from build123d import *

# Parameters (mm, degrees)
SKETCH1_W               = 96
SKETCH1_H               = 185
PLATE_DEPTH             = 5
STANDOFF_HOLES_REACH    = 106.332
SKETCH2_R               = 1.7
POWER_BOARD_HOLES_REACH = 106.332
SKETCH3_R               = 1.7
FILLET1_R               = 1
M2_5_CLEARANCE_HOLE1_D  = 2.9
M3_CLEARANCE_HOLE2_D    = 3.4
CUT_EXTRUDE1_REACH      = 106.332


with BuildPart() as part:
    # Sketch1 → plate (new body)
    with BuildSketch(Plane(origin=(0, 0, 0), x_dir=(1, 0, 0), z_dir=(0, 1, 0))):
        Rectangle(SKETCH1_W, SKETCH1_H)
    extrude(amount=PLATE_DEPTH)

    # Sketch2 → standoff-holes (cut, up to next)
    with BuildSketch(Plane(origin=(0, 5, 0), x_dir=(1, 0, 0), z_dir=(0, 1, 0)), mode=Mode.PRIVATE) as standoff_holes_sk1:
        with Locations(Location((44, 74, 0), (0, 0, 270))):
            Circle(SKETCH2_R)
    standoff_holes_tool1 = extrude(standoff_holes_sk1.sketch, amount=-STANDOFF_HOLES_REACH, mode=Mode.PRIVATE) & part.part
    # Sketch2 → standoff-holes (cut, up to next)
    with BuildSketch(Plane(origin=(0, 5, 0), x_dir=(1, 0, 0), z_dir=(0, 1, 0)), mode=Mode.PRIVATE) as standoff_holes_sk2:
        with Locations(Location((-44, 74, 0), (0, 0, 270))):
            Circle(SKETCH2_R)
    standoff_holes_tool2 = extrude(standoff_holes_sk2.sketch, amount=-STANDOFF_HOLES_REACH, mode=Mode.PRIVATE) & part.part
    # Sketch2 → standoff-holes (cut, up to next)
    with BuildSketch(Plane(origin=(0, 5, 0), x_dir=(1, 0, 0), z_dir=(0, 1, 0)), mode=Mode.PRIVATE) as standoff_holes_sk3:
        with Locations(Location((44, -74, 0), (0, 0, 270))):
            Circle(SKETCH2_R)
    standoff_holes_tool3 = extrude(standoff_holes_sk3.sketch, amount=-STANDOFF_HOLES_REACH, mode=Mode.PRIVATE) & part.part
    # Sketch2 → standoff-holes (cut, up to next)
    with BuildSketch(Plane(origin=(0, 5, 0), x_dir=(1, 0, 0), z_dir=(0, 1, 0)), mode=Mode.PRIVATE) as standoff_holes_sk4:
        with Locations(Location((-44, -74, 0), (0, 0, 270))):
            Circle(SKETCH2_R)
    standoff_holes_tool4 = extrude(standoff_holes_sk4.sketch, amount=-STANDOFF_HOLES_REACH, mode=Mode.PRIVATE) & part.part
    add(standoff_holes_tool1.solids().sort_by_distance((44, 5, -74))[0], mode=Mode.SUBTRACT)
    add(standoff_holes_tool2.solids().sort_by_distance((-44, 5, -74))[0], mode=Mode.SUBTRACT)
    add(standoff_holes_tool3.solids().sort_by_distance((44, 5, 74))[0], mode=Mode.SUBTRACT)
    add(standoff_holes_tool4.solids().sort_by_distance((-44, 5, 74))[0], mode=Mode.SUBTRACT)

    # Sketch3 → power-board-holes (cut, up to next)
    with BuildSketch(Plane(origin=(0, 5, 0), x_dir=(1, 0, 0), z_dir=(0, 1, 0)), mode=Mode.PRIVATE) as power_board_holes_sk1:
        with Locations(Location((38, 0, 0), (0, 0, 270))):
            Circle(SKETCH3_R)
    power_board_holes_tool1 = extrude(power_board_holes_sk1.sketch, amount=-POWER_BOARD_HOLES_REACH, mode=Mode.PRIVATE) & part.part
    # Sketch3 → power-board-holes (cut, up to next)
    with BuildSketch(Plane(origin=(0, 5, 0), x_dir=(1, 0, 0), z_dir=(0, 1, 0)), mode=Mode.PRIVATE) as power_board_holes_sk2:
        with Locations(Location((-38, 0, 0), (0, 0, 270))):
            Circle(SKETCH3_R)
    power_board_holes_tool2 = extrude(power_board_holes_sk2.sketch, amount=-POWER_BOARD_HOLES_REACH, mode=Mode.PRIVATE) & part.part
    add(power_board_holes_tool1.solids().sort_by_distance((38, 5, 0))[0], mode=Mode.SUBTRACT)
    add(power_board_holes_tool2.solids().sort_by_distance((-38, 5, 0))[0], mode=Mode.SUBTRACT)

    # Fillet1
    fillet1_edges = [part.edges().sort_by_distance(p)[0] for p in [
        (48, 2.5, 92.5),
        (-48, 2.5, 92.5),
        (-48, 2.5, -92.5),
        (48, 2.5, -92.5),
    ]]
    fillet(fillet1_edges, radius=FILLET1_R)

    # M2.5 Clearance Hole1 (through all)
    with Locations(Plane(origin=(0, 5, 0), x_dir=(1, 0, 0), z_dir=(0, 1, 0))):
        with Locations((-39, -85.98), (19, -85.98), (-39, -36.98), (19, -36.98)):
            Hole(M2_5_CLEARANCE_HOLE1_D / 2)

    # M3 Clearance Hole2 (through all)
    with Locations(Plane(origin=(0, 5, 0), x_dir=(1, 0, 0), z_dir=(0, 1, 0))):
        with Locations((-39.49999847, 79.47999944), (-39.49999847, 37.47999962), (39.50000101, 37.47999962), (39.50000101, 79.47999944)):
            Hole(M3_CLEARANCE_HOLE2_D / 2)

    # Sketch12 → Cut-Extrude1 (cut, up to next)
    with BuildSketch(Plane(origin=(0, 5, 0), x_dir=(1, 0, 0), z_dir=(0, 1, 0)), mode=Mode.PRIVATE) as cut_extrude1_sk1:
        with BuildLine():
            Line((-25, -27), (25, -27))
            ThreePointArc((25, -27), (28, -30), (25, -33))
            Line((25, -33), (-25, -33))
            ThreePointArc((-25, -33), (-28, -30), (-25, -27))
        make_face()
    cut_extrude1_tool1 = extrude(cut_extrude1_sk1.sketch, amount=-CUT_EXTRUDE1_REACH, mode=Mode.PRIVATE) & part.part
    add(cut_extrude1_tool1.solids().sort_by_distance((0, 5, 30))[0], mode=Mode.SUBTRACT)


solid = part.part
Design review of the part built by this model. Coordinates are the model's own, in mm. A direction names the side the tool comes from. Coordinates: 2 decimals unless noted, no trailing zeros. Loops run counter-clockwise (first coordinate to the right, second up) from the corner with the lowest first, then second, coordinate; pieces in that order, holes last.
Item 1: Add section C-C (z = 74). Write out the cut boundary in (x, y).
Completed:
outline: (-48, 0) - (-45.7, 0) - (-45.7, 5) - (-48, 5) - close; (-42.3, 0) - (42.3, 0) - (42.3, 5) - (-42.3, 5) - close; (45.7, 0) - (48, 0) - (48, 5) - (45.7, 5) - close
Item 2: For faces 1 (the flat face through (0, 3, 27)), 2 (the flat face through (48, 2, 1)), list the 3-axis set-ups (+Z, -Z, +X, -X, +Y, -Y) from which the entire face can be reached by the end or side of a thin tool; tool diameter is ignored.
Completed:
face 1: +Y, -Y
face 2: +Z, -Z, +X, +Y, -Y
Item 3: Add section D-D (y = 0.9). Give the number of separate pieces and of enclosed holes in the cut face, and give its area (3 significant figures).
Completed:
separate pieces: 1
enclosed holes: 15
area: 17,300 mm2
Item 4: Add section B-B (z = 30). Write out the cut boundary in (x, y).
Completed:
outline: (-48, 0) - (-28, 0) - (-28, 5) - (-48, 5) - close; (28, 0) - (48, 0) - (48, 5) - (28, 5) - close
Item 5: Add section A-A (x = 9). Write out the cut boundary in (y, z).
Completed:
outline: (0, -92.5) - (5, -92.5) - (5, 27) - (0, 27) - close; (0, 33) - (5, 33) - (5, 92.5) - (0, 92.5) - close
Item 6: Draft analysis for pull direction Z (two halves, no side actions). For faces 3 (the cylindrical face through (44.07, 2.54, 72.3)), 4 (the flat face through (-1, 2, 92.5)), 5 (the flat face through (-48, 2, 1)), state which applies: pulls with the +Z half, pulls with the -Z half, needs draft (parallel to the pull), parting line crosses it, or undercut.
Completed:
face 3: undercut
face 4: pulls with the +Z half
face 5: needs draft
Item 7: Wall thickness on L1, parallel to X at y = 1.5, z = 0; L2, parallel to Z at x = 19, y = 2.15; L3, parallel to Z at x = 0, y = 2.9: over which ranges is each line inside the solid? List them lowest first.
Completed:
L1: x = -48 to -39.7, -36.3 to 36.3, 39.7 to 48
L2: z = -92.5 to 27, 33 to 35.53, 38.43 to 84.53, 87.43 to 92.5
L3: z = -92.5 to 27, 33 to 92.5
